Here's how the part is built. I have some questions about the finished solid (model axes, mm). A direction names the side the tool comes from. Coordinates: 2 decimals unless noted, no trailing zeros. Write each loop counter-clockwise with the first axis right and the second up, starting at its lowest first coordinate (ties: lowest second). Pieces come first, ordered by that corner, then holes.
(1) Which directions (+Z, -Z, +X, -X, +Y, -Y) give clear straight access to the entire face, cutting with the end or side of a thin tool? Please do faces 1 (the flat face through (-31.41, -0.28, -10.94)), 2 (the cylindrical face through (29.14, -0.28, 19.39)), 3 (the flat face through (-14.477, -0.28, -29.95)).
(2) Thinking about a two-plate mould opening in X: for faces 4 (the cylindrical face through (-34.314, -0.28, 6.894)), 5 (the cylindrical face through (29.064, -0.28, -19.501)), 6 (the cylindrical face through (26.093, -0.28, -10.84)), which applies, released by +X, released by -X, zero draft, split by the parting line, or undercut?
(3) Imagine slicing it at A-A, the plane x = 0. List the corners of the cut face in (y, z) for me, plus the area to 3 significant figures.
(4) Imagine slicing it at B-B, the plane z = -7. List the corners of the cut face in (x, y) for me, plus the area to 3 significant figures.
(5) For pin 1 Ø12 at (y, z) = (-8.5, 14) entering from +X; pin 2 Ø3 at (x, z) = (0, 30.12) entering from -Y; pin 3 Ø6 at (y, z) = (8, -7) entering from +X; pin 4 Ø10 at (y, z) = (-11.5, -11.5) entering from +X, each with a flat end and sliding along its axis, tell me the tip position at first contact or that it passes through.
(6) Please list where these lines run through material, in increasing order: probe 1 along Z at (x, y) = (21.5, 10.5); probe 2 along X at (y, z) = (13, 21); probe 3 along X at (y, z) = (-11, -22).
```python
from build123d import *

# Parameters (mm, degrees)
F1_DEPTH = 20


# Not quite as in the source:
# - ends of sketch curves that miss each other by under 0.0002 mm in the source are joined


with BuildPart() as f1:
    # F0 (on Front) → F1 (new body, symmetric)
    with BuildSketch(Plane.XZ):
        with BuildLine():
            Line((34.9101450984, 2.4936542119), (34.9110309298, 2.4939766282))
            ThreePointArc((34.9110309298, 2.4939766282), (34.3286939173, 6.8220798831), (33.2119055423, 11.0439725756))
            Line((33.2119055423, 11.0439725756), (29.5663055038, 10.8358313755))
            ThreePointArc((29.5663055038, 10.8358313755), (26.0913542461, 10.8432258269), (28.6289762641, 13.2172130666))
            Line((28.6289762641, 13.2172130666), (31.2984883804, 15.6633702382))
            Line((31.2984883804, 15.6633702382), (31.2991833986, 15.6640071049))
            ThreePointArc((31.2991833986, 15.6640071049), (29.1048807425, 19.4398023901), (26.457454434, 22.9129462285))
            Line((26.457454434, 22.9129462285), (23.1690113636, 21.3255380981))
            ThreePointArc((23.1690113636, 21.3255380981), (19.9557452862, 20.0025634058), (21.3917167446, 23.1669475309))
            Line((21.3917167446, 23.1669475309), (22.9219205281, 26.4484801345))
            Line((22.9219205281, 26.4484801345), (22.9223189227, 26.4493344946))
            ThreePointArc((22.9223189227, 26.4493344946), (19.450113311, 29.0979912054), (15.6750957256, 31.2936315245))
            Line((15.6750957256, 31.2936315245), (13.2444452709, 28.5686249618))
            ThreePointArc((13.2444452709, 28.5686249618), (10.7820550057, 26.1166920299), (10.897762267, 29.5897242426))
            Line((10.897762267, 29.5897242426), (11.055698063, 33.2070486864))
            Line((11.055698063, 33.2070486864), (11.0557391823, 33.2079904712))
            ThreePointArc((11.0557391823, 33.2079904712), (6.8342424437, 34.3262746336), (2.5063457881, 34.9101450984))
            Line((2.5063457881, 34.9101450984), (1.3035324469, 31.4623976502))
            ThreePointArc((1.3035324469, 31.4623976502), (-0.0331054099, 28.2547910408), (-1.2552777272, 31.5077336698))
            Line((-1.2552777272, 31.5077336698), (-2.4936542119, 34.9101450984))
            Line((-2.4936542119, 34.9101450984), (-2.4939766282, 34.9110309298))
            ThreePointArc((-2.4939766282, 34.9110309298), (-6.8220798831, 34.3286939173), (-11.0439725756, 33.2119055423))
            Line((-11.0439725756, 33.2119055423), (-10.8358313755, 29.5663055038))
            ThreePointArc((-10.8358313755, 29.5663055038), (-10.8432258269, 26.0913542461), (-13.2172130666, 28.6289762641))
            Line((-13.2172130666, 28.6289762641), (-15.6633702382, 31.2984883804))
            Line((-15.6633702382, 31.2984883804), (-15.6640071049, 31.2991833986))
            ThreePointArc((-15.6640071049, 31.2991833986), (-19.4398023901, 29.1048807425), (-22.9129462285, 26.457454434))
            Line((-22.9129462285, 26.457454434), (-21.3255380981, 23.1690113636))
            ThreePointArc((-21.3255380981, 23.1690113636), (-20.0014808321, 19.9567910089), (-23.1670922293, 21.3887099076))
            Line((-23.1670922293, 21.3887099076), (-23.3543714527, 21.4791139546))
            Line((-23.3543714527, 21.4791139546), (-26.4484801345, 22.9219205281))
            Line((-26.4484801345, 22.9219205281), (-26.4493344946, 22.9223189227))
            ThreePointArc((-26.4493344946, 22.9223189227), (-29.0979912054, 19.450113311), (-31.2936315245, 15.6750957256))
            Line((-31.2936315245, 15.6750957256), (-28.5686249618, 13.2444452709))
            ThreePointArc((-28.5686249618, 13.2444452709), (-26.1166920299, 10.7820550057), (-29.5897242426, 10.897762267))
            Line((-29.5897242426, 10.897762267), (-33.2070486864, 11.055698063))
            Line((-33.2070486864, 11.055698063), (-33.2079904712, 11.0557391823))
            ThreePointArc((-33.2079904712, 11.0557391823), (-34.3262746336, 6.8342424437), (-34.9101450984, 2.5063457881))
            Line((-34.9101450984, 2.5063457881), (-31.4623976502, 1.3035324469))
            ThreePointArc((-31.4623976502, 1.3035324469), (-29.3324543071, 1.6932130885), (-28.2642048894, -0.1902286623))
            ThreePointArc((-28.2642048894, -0.1902286623), (-29.4892446104, -1.8074791131), (-31.4669238904, -1.3547032257))
            Line((-31.4669238904, -1.3547032257), (-34.9066388382, -2.5547142739))
            ThreePointArc((-34.9066388382, -2.5547142739), (-34.3227460841, -6.8519414215), (-33.2119055423, -11.0439725756))
            Line((-33.2119055423, -11.0439725756), (-29.5663055038, -10.8358313755))
            ThreePointArc((-29.5663055038, -10.8358313755), (-26.0913542461, -10.8432258269), (-28.6289762641, -13.2172130666))
            Line((-28.6289762641, -13.2172130666), (-31.2984883804, -15.6633702382))
            Line((-31.2984883804, -15.6633702382), (-31.2991833986, -15.6640071049))
            ThreePointArc((-31.2991833986, -15.6640071049), (-29.1048807425, -19.4398023901), (-26.457454434, -22.9129462285))
            Line((-26.457454434, -22.9129462285), (-23.1867866645, -21.3341186503))
            ThreePointArc((-23.1867866645, -21.3341186503), (-19.9778704256, -19.9570429396), (-21.3046655311, -23.1870732319))
            Line((-21.3046655311, -23.1870732319), (-22.8920736615, -26.4755163023))
            ThreePointArc((-22.8920736615, -26.4755163023), (-19.4334813455, -29.1091017174), (-15.6750957256, -31.2936315245))
            Line((-15.6750957256, -31.2936315245), (-13.2444452709, -28.5686249618))
            ThreePointArc((-13.2444452709, -28.5686249618), (-10.7820550057, -26.1166920299), (-10.897762267, -29.5897242426))
            Line((-10.897762267, -29.5897242426), (-11.055698063, -33.2070486864))
            Line((-11.055698063, -33.2070486864), (-11.0557391823, -33.2079904712))
            ThreePointArc((-11.0557391823, -33.2079904712), (-6.8342424437, -34.3262746336), (-2.5063457881, -34.9101450984))
            Line((-2.5063457881, -34.9101450984), (-1.3035324469, -31.4623976502))
            ThreePointArc((-1.3035324469, -31.4623976502), (-1.3388311966, -28.8194805066), (1.3040932823, -28.7847353157))
            ThreePointArc((1.3040932823, -28.7847353157), (1.8690592706, -30.1571657006), (1.2555114416, -31.5085763676))
            Line((1.2555114416, -31.5085763676), (2.4936542119, -34.9101450984))
            Line((2.4936542119, -34.9101450984), (2.4939766282, -34.9110309298))
            ThreePointArc((2.4939766282, -34.9110309298), (6.8220798831, -34.3286939173), (11.0439725756, -33.2119055423))
            Line((11.0439725756, -33.2119055423), (10.8358313755, -29.5663055038))
            ThreePointArc((10.8358313755, -29.5663055038), (10.8432258269, -26.0913542461), (13.2172130666, -28.6289762641))
            Line((13.2172130666, -28.6289762641), (15.6633702382, -31.2984883804))
            Line((15.6633702382, -31.2984883804), (15.6640071049, -31.2991833986))
            ThreePointArc((15.6640071049, -31.2991833986), (19.4283242222, -29.112543996), (22.8920736615, -26.4755163023))
            Line((22.8920736615, -26.4755163023), (21.3046655311, -23.1870732319))
            ThreePointArc((21.3046655311, -23.1870732319), (19.9999615902, -19.9356459921), (23.1847053682, -21.3955906956))
            Line((23.1847053682, -21.3955906956), (23.6096103837, -21.5981338228))
            Line((23.6096103837, -21.5981338228), (26.4484801345, -22.9219205281))
            Line((26.4484801345, -22.9219205281), (26.4493344946, -22.9223189227))
            ThreePointArc((26.4493344946, -22.9223189227), (29.0979912054, -19.450113311), (31.2936315245, -15.6750957256))
            Line((31.2936315245, -15.6750957256), (28.5686249618, -13.2444452709))
            ThreePointArc((28.5686249618, -13.2444452709), (26.1166920299, -10.7820550057), (29.5897242426, -10.897762267))
            Line((29.5897242426, -10.897762267), (33.2070486864, -11.055698063))
            Line((33.2070486864, -11.055698063), (33.2079904712, -11.0557391823))
            ThreePointArc((33.2079904712, -11.0557391823), (34.3215316909, -6.8580217548), (34.9066388382, -2.5547142739))
            Line((34.9066388382, -2.5547142739), (31.4669238904, -1.3547032257))
            ThreePointArc((31.4669238904, -1.3547032257), (29.4892446104, -1.8074791131), (28.2642048894, -0.1902286623))
            ThreePointArc((28.2642048894, -0.1902286623), (29.3625733997, 1.7069569752), (31.5077336698, 1.2552777272))
            Line((31.5077336698, 1.2552777272), (34.9101450984, 2.4936542119))
        make_face()
    extrude(amount=F1_DEPTH, both=True)


solid = f1.part
```
Recorded:
1. face 1: +Y, -Y
1. face 2: +Z, +X, +Y, -Y
1. face 3: -Z, +Y, -Y
2. face 4: released by -X
2. face 5: released by +X
2. face 6: undercut
3. outline: (-20, -28.25) - (20, -28.25) - (20, 28.25) - (-20, 28.25) - close
3. area: 2,260 mm2
4. outline: (-34.29, -20) - (34.29, -20) - (34.29, 20) - (-34.29, 20) - close
4. area: 2,740 mm2
5. pin 1: stops at x = 34.07
5. pin 2: passes through
5. pin 3: stops at x = 34.77
5. pin 4: stops at x = 34.39
6. probe 1: z = -27.62 to -23.59, -19.43 to 19.44, 23.4 to 27.62
6. probe 2: x = -28 to -23.14, -19.46 to 19.46, 23.14 to 28
6. probe 3: x = -27.22 to -24.57, -19.55 to 19.55, 24.47 to 27.22
